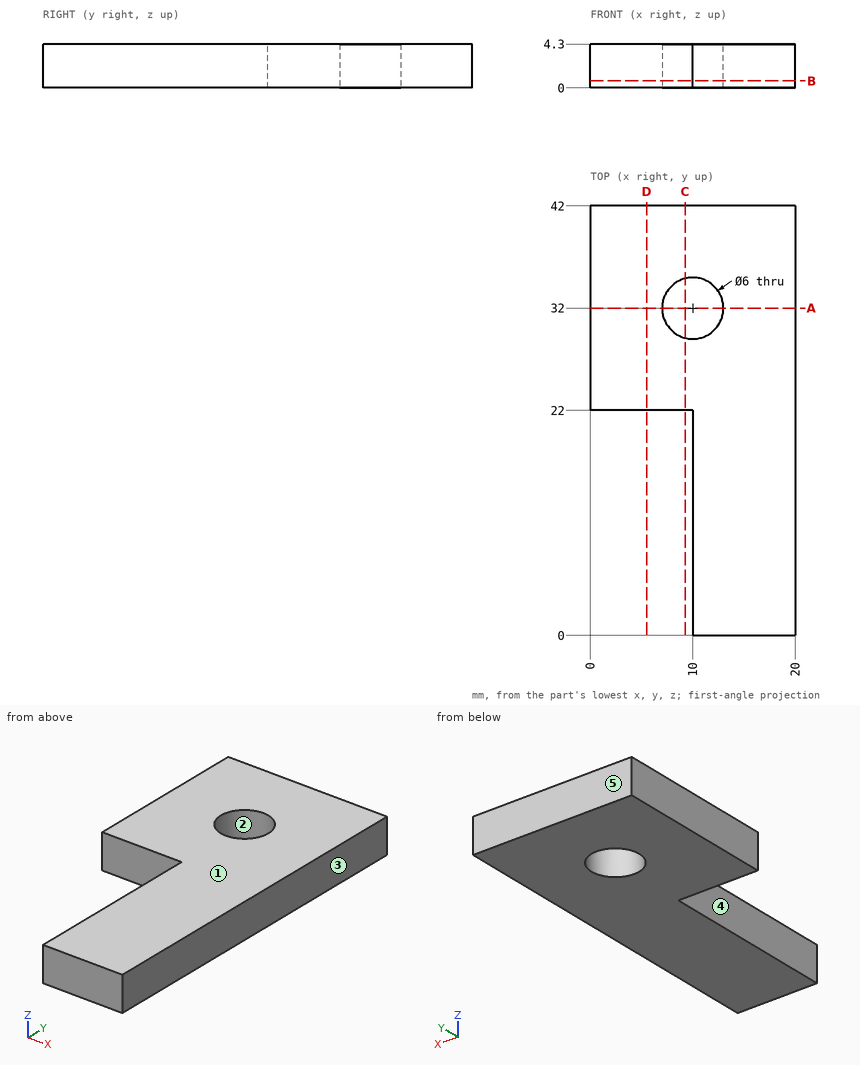
Design review of the part shown in the three views and the two pictorial views. Dimensions are in mm from the part's minimum x, y and z. A direction names the side the tool comes from. Round coordinates to 2 decimals unless told otherwise and drop trailing zeros. Write each loop counter-clockwise with the first axis right and the second up, starting at its lowest first coordinate (ties: lowest second). Pieces come first, ordered by that corner, then holes. Notation, with made-up numbers: (68, 65) - (109, 65) arc R21 cw to (109, 100) - close; hole circle Ø7 at (-13, -38). An arc over 180 degrees is marked (long way). Return JSON: item names as keys, results as strings. Group by question number.
Item 1: We need section B-B on z = 0.7. Write out the cut boundary in (x, y), and give its area (3 significant figures).
Item 2: We need section A-A on y = 32. Write out the cut boundary in (x, z).
Item 3: The part is to be moulded in two halves that separate along X. For the marked faces 1, 2 and 3, say which applies: pulls with the +X half, pulls with the -X half, needs draft (parallel to the pull), parting line crosses it, or undercut.
Item 4: We need section D-D on x = 5.5. Write out the cut boundary in (y, z), and give its area (3 significant figures).
Item 5: Insertion check: P1, Ø3.5, axis at x = 10, y = 32, coming from the +Z side. The pin has a flat end and moves straight along its axis. Give the tip position at first contact, or say it passes through.
Item 6: Machinability: for the marked faces 4 and 5, which of the approach directions +Z, -Z, +X, -X, +Y, -Y give a long, thin tool a straight path to every point of the face, cutting with its end or side? Answer none if there is none.
Item 7: We need section C-C on x = 9.25. Write out the cut boundary in (y, z), and give its area (3 significant figures).
Item 8: For probe 1 along X at (y, z) = (9, 1.5); probe 2 along Y at (x, z) = (3.75, 2); probe 3 along X at (y, z) = (33, 1.2), list the stretches that pass through material, from the lowest coordinate up. Write a range as [from, to].
Model answer:
{
 "1": {"outline": "(0, 22) - (10, 22) - (10, 0) - (20, 0) - (20, 42) - (0, 42) - close; hole circle Ø6 at (10, 32)", "area": "592 mm²"},
 "2": {"outline": "(0, 0) - (7, 0) - (7, 4.3) - (0, 4.3) - close; (13, 0) - (20, 0) - (20, 4.3) - (13, 4.3) - close"},
 "3": {"face 1": "needs draft", "face 2": "undercut", "face 3": "pulls with the +X half"},
 "4": {"outline": "(22, 0) - (42, 0) - (42, 4.3) - (22, 4.3) - close", "area": "86.0 mm²"},
 "5": {"P1": "passes through"},
 "6": {"face 4": "+Z, -Z, -X, -Y", "face 5": "+Z, -Z, +X, -X, +Y"},
 "7": {"outline": "(22, 0) - (29.1, 0) - (29.1, 4.3) - (22, 4.3) - close; (34.9, 0) - (42, 0) - (42, 4.3) - (34.9, 4.3) - close", "area": "61.0 mm²"},
 "8": {"probe 1": "x = [10, 20]", "probe 2": "y = [22, 42]", "probe 3": "x = [0, 7.17], [12.83, 20]"}
}
